Print and shaded views of the part. All mm, measured from the part's lowest x, y and z. A direction names the side the tool comes from. Round coordinates to 2 decimals unless told otherwise and drop trailing zeros. Loops run counter-clockwise (first coordinate to the right, second up) from the corner with the lowest first, then second, coordinate; pieces in that order, holes last. Notation, with made-up numbers: (31.5, 56.25) - (42.5, 56.25) arc R23 ccw to (42.5, 80.25) - close; hole circle Ø2 at (28, 0). An arc over 180 degrees is marked (long way). Answer as a JSON object with one key per item and string values.
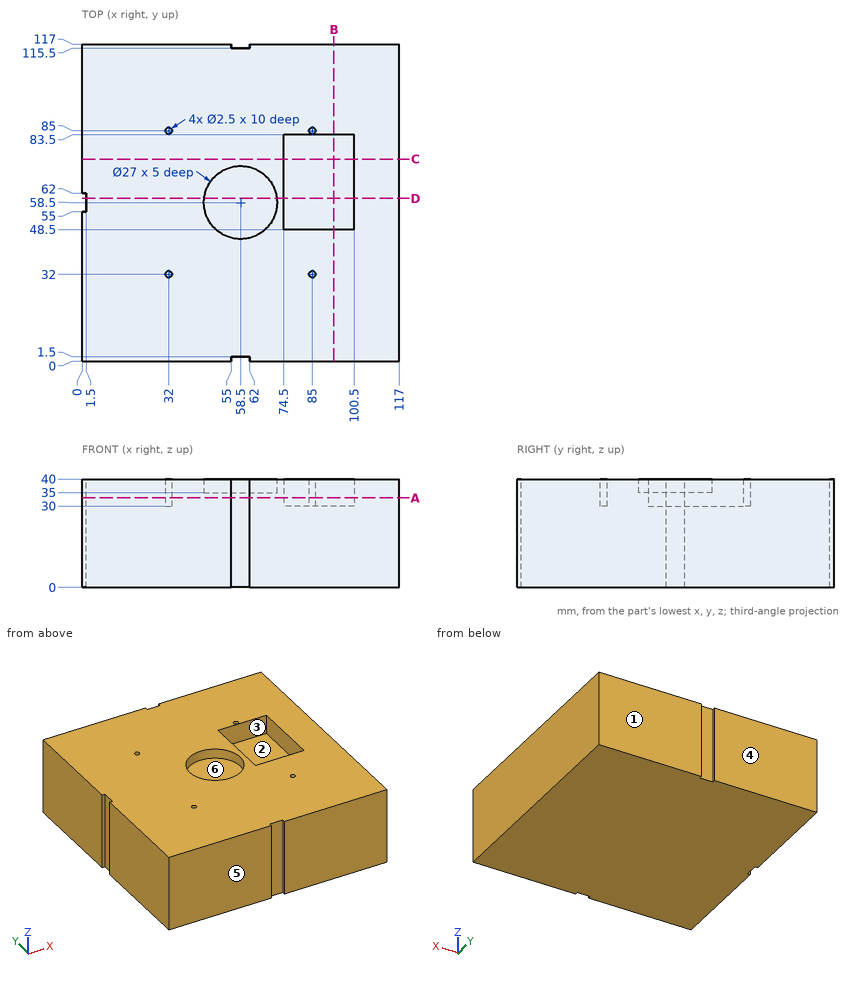
1) Slice it at B-B on x = 93. List the corners of the cut face in (y, z), then the cut area to 3 significant figures.
Values follow:
{"outline": "(0, 0) - (117, 0) - (117, 40) - (83.5, 40) - (83.5, 30) - (48.5, 30) - (48.5, 40) - (0, 40) - close", "area": "4,330 mm²"}
2) Slice it at A-A on z = 33. List the corners of the cut face in (x, y).
Values follow:
{"outline": "(0, 0) - (55, 0) - (55, 1.5) - (62, 1.5) - (62, 0) - (117, 0) - (117, 117) - (62, 117) - (62, 115.5) - (55, 115.5) - (55, 117) - (0, 117) - (0, 62) - (1.5, 62) - (1.5, 55) - (0, 55) - close; hole circle Ø2.5 at (32, 32); hole circle Ø2.5 at (32, 85); hole (74.5, 48.5) - (100.5, 48.5) - (100.5, 83.5) - (74.5, 83.5) - close; hole circle Ø2.5 at (85, 32); hole circle Ø2.5 at (85, 85)"}
3) Drop flat-ended pins along their axis: P1, Ø2, axis at x = 85, y = 32, coming from the +Z side; P2, Ø6, axis at x = 36.5, z = 31, coming from the -Y side; P3, Ø5, axis at y = 58.5, z = 37, coming from the -X side; P4, Ø3.5, axis at x = 57.5, z = 24, coming from the +Y side. Give the stop position or say it passes through.
Values follow:
{"P1": "z = 30", "P2": "y = 0", "P3": "x = 1.5", "P4": "y = 115.5"}
4) Probe probe 1 along Y at (x, z) = (85, 32); probe 2 along Y at (x, z) = (32, 37.75); probe 3 along X at (y, z) = (61, 31.5). List the from-to ranges inside material, lowest first.
Values follow:
{"probe 1": "0 to 30.75, 33.25 to 48.5, 83.5 to 83.75, 86.25 to 117", "probe 2": "0 to 30.75, 33.25 to 83.75, 86.25 to 117", "probe 3": "1.5 to 74.5, 100.5 to 117"}
5) Two-plate mould, pull along Y, no slides. Class the marked faces 3, 4, 5 and 6: pulls with the +Y half, pulls with the -Y half, needs draft (parallel to the pull), parting line crosses it, or undercut.
Values follow:
{"face 3": "undercut", "face 4": "pulls with the +Y half", "face 5": "pulls with the -Y half", "face 6": "undercut"}
6) Slice it at D-D on y = 60. List the corners of the cut face in (x, z).
Values follow:
{"outline": "(1.5, 0) - (117, 0) - (117, 40) - (100.5, 40) - (100.5, 30) - (74.5, 30) - (74.5, 40) - (71.92, 40) - (71.92, 35) - (45.08, 35) - (45.08, 40) - (1.5, 40) - close"}
7) Slice it at C-C on y = 74.5. List the corners of the cut face in (x, z).
Values follow:
{"outline": "(0, 0) - (117, 0) - (117, 40) - (100.5, 40) - (100.5, 30) - (74.5, 30) - (74.5, 40) - (0, 40) - close"}
8) Tool access for the marked faces 1 and 2: list every direction of +Z, -Z, +X, -X, +Y, -Y with a clear straight run to the whole face (end or side of a thin tool).
Values follow:
{"face 1": "+Z, -Z, +X, -X, +Y", "face 2": "+Z"}
